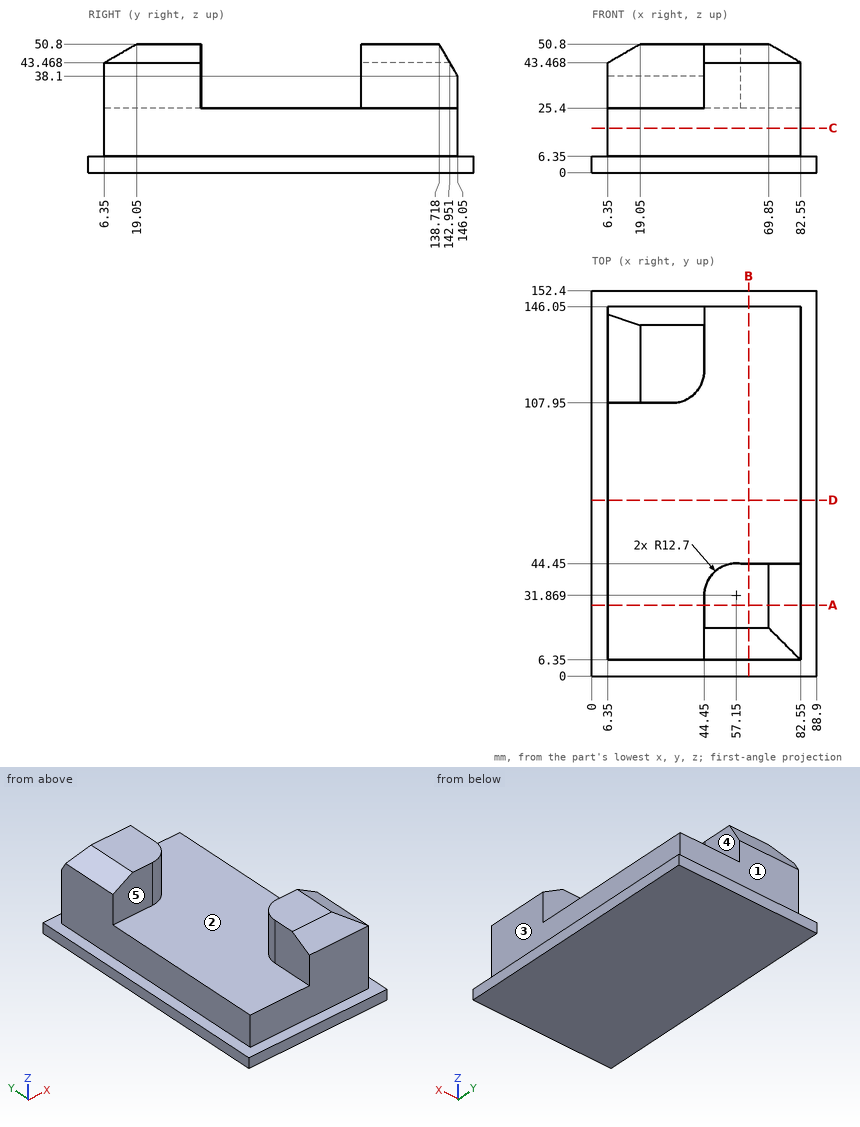
Geometry check sheet. Reference: drawing and pictorial views, mm from the part's lowest x, y, z. A direction names the side the tool comes from. Round coordinates to 2 decimals unless told otherwise and drop trailing zeros. Loops run counter-clockwise (first coordinate to the right, second up) from the corner with the lowest first, then second, coordinate; pieces in that order, holes last. Notation, with made-up numbers: (14, 27.5) - (73, 27.5) arc R16 cw to (73, 33.5) - close; hole circle Ø2 at (66, -21). An arc over 180 degrees is marked (long way). One line per question, with ' | ' between items. Start each with the question number.
1. Cross-section at C-C on z = 17.5. Record the cut outline in (x, y).
2. Scan lines: line 1 (Z direction, x = 28.5, y = 50.5); line 2 (Y direction, x = 14, z = 35.5); line 3 (Y direction, x = 63, z = 26). Record each from-to range of solid material in increasing order. Write a range as [from, to].
3. Cross-section at A-A on y = 28. Record the cut outline in (x, z), then the cut area to 3 significant figures.
4. Cross-section at B-B on x = 62. Record the cut outline in (y, z), then the cut area to 3 significant figures.
5. Tool access check on the marked faces 1, 2, 3, 4 and 5. Record the directions out of +Z, -Z, +X, -X, +Y, -Y that give a thin tool (end or side, any length) a straight path to the whole face; none if there is none.
6. Cross-section at D-D on y = 69.5. Record the cut outline in (x, z).
7. Depth check by flat-ended pin: pin 1 (6 mm diameter, centred on x = 55, z = 30.5, fed in from -Y); pin 2 (7.5 mm diameter, centred on x = 13.5, z = 32, fed in from -Y); pin 3 (1 mm diameter, centred on x = 58.5, y = 17, fed in from +Z) (1 decimal); pin 4 (12 mm diameter, centred on y = 51.5, z = 32, fed in from +X). Enter the tip coordinate at first touch or a pass-through.
Taken from the geometry:
1) outline: (6.35, 6.35) - (82.55, 6.35) - (82.55, 146.05) - (6.35, 146.05) - close
2) line 1: [0, 25.4] | line 2: [107.95, 146.05] | line 3: [6.35, 44.45]
3) outline: (0, 0) - (88.9, 0) - (88.9, 6.35) - (82.55, 6.35) - (82.55, 43.47) - (69.85, 50.8) - (44.45, 50.8) - (44.45, 25.4) - (6.35, 25.4) - (6.35, 6.35) - (0, 6.35) - close | area: 2,940 mm²
4) outline: (0, 0) - (152.4, 0) - (152.4, 6.35) - (146.05, 6.35) - (146.05, 25.4) - (44.45, 25.4) - (44.45, 50.8) - (19.05, 50.8) - (6.35, 43.47) - (6.35, 6.35) - (0, 6.35) - close | area: 4,550 mm²
5) face 1: +Z, +X, -X, +Y | face 2: +Z | face 3: +Z, +X, +Y, -Y | face 4: +Z, +X, +Y | face 5: +Z, +X, -X, -Y
6) outline: (0, 0) - (88.9, 0) - (88.9, 6.35) - (82.55, 6.35) - (82.55, 25.4) - (6.35, 25.4) - (6.35, 6.35) - (0, 6.35) - close
7) pin 1: y = 6.35 | pin 2: y = 107.95 | pin 3: z = 49.9 | pin 4: through
